from build123d import *

# Parameters (mm, degrees)
SKETCH_1_R          = 1.5000000000000002
EXTRUDE_1_DEPTH     = 10
EXTRUDE_START       = 1
SKETCH_2_R          = 2.75
SKETCH_2_R_2        = 1.5000000000000002
EXTRUDE_2_DEPTH     = 1
SKETCH_3_R          = 2.75
SKETCH_3_R_2        = 1.5000000000000002
EXTRUDE_3_DEPTH     = 1
SKETCH_5_R          = 6.5
EXTRUDE_4_DEPTH     = 18
SKETCH_7_R          = 4.499999999999999
CUT_EXTRUDE_1_DEPTH = 18
SKETCH_9_R          = 2.8700119692288277
SKETCH_12_W         = 5.249259279764373
SKETCH_12_H         = 2.7755664511126334
SKETCH_12_H_2       = 2.7755664511126383
EXTRUDE_5_DEPTH     = 5
CUT_EXTRUDE_2_DEPTH = 20


with BuildPart() as part:
    # 草图1 → 凸台-拉伸1 (new body)
    with BuildSketch(Plane.XY):
        with BuildLine():
            Line((-2.75, 0), (-2.7500000000000004, 9.5))
            Line((-2.7500000000000004, 9.5), (2.7500000000000004, 9.5))
            Line((2.7500000000000004, 9.5), (2.75, 0))
            ThreePointArc((2.75, 0), (-5.1e-16, -2.75), (-2.75, 0))
        make_face()
        Circle(SKETCH_1_R, mode=Mode.SUBTRACT)
    extrude(amount=EXTRUDE_1_DEPTH)

    # 草图2 → 凸台-拉伸2 (add)
    with BuildSketch(Plane(origin=(0, 0, 0), x_dir=(-1, 0, 0), z_dir=(0, 0, -1)).offset(EXTRUDE_START)):
        Circle(SKETCH_2_R)
        Circle(SKETCH_2_R_2, mode=Mode.SUBTRACT)
    extrude(amount=-EXTRUDE_2_DEPTH)

    # 草图3 → 凸台-拉伸3 (add)
    with BuildSketch(Plane.XY.offset(10)):
        with Locations(Location((0, 0, 0), (0, 0, 180))):
            Circle(SKETCH_3_R)
        with Locations(Location((0, 0, 0), (0, 0, 180))):
            Circle(SKETCH_3_R_2, mode=Mode.SUBTRACT)
    extrude(amount=EXTRUDE_3_DEPTH)

    # 草图5 → 凸台-拉伸4 (add)
    with BuildSketch(Plane.ZY.offset(4.75)):
        with Locations(Location((5, 13.164932727725386, 0), (0, 0, 270))):
            Circle(SKETCH_5_R)
    extrude(amount=-EXTRUDE_4_DEPTH)

    # 草图7 → 切除-拉伸1 (cut)
    with BuildSketch(Plane.ZY.offset(4.75)):
        with Locations(Location((5, 13.164932727725386, 0), (0, 0, 270))):
            Circle(SKETCH_7_R)
    extrude(amount=-CUT_EXTRUDE_1_DEPTH, mode=Mode.SUBTRACT)

    # 扫描2: sweep along a path in 草图11
    with BuildLine(Plane(origin=(0, 0, 5), x_dir=(-1, 0, 0), z_dir=(0, 0, -1))) as sweep_2_path:
        Line((-7, 24), (0, 19))
    # 草图9 → 扫描2 (sweep)
    with BuildSketch(Plane(origin=(0, 19, 0), x_dir=(1, 0, 0), z_dir=(0, 1, 0))):
        with Locations((-0.00737750074134282, -4.885467390073623)):
            Circle(SKETCH_9_R)
    sweep(path=sweep_2_path.line)

    # 草图12 → 凸台-拉伸5 (add)
    with BuildSketch(Plane(origin=(0, 19, 0), x_dir=(1, 0, 0), z_dir=(0, 1, 0))):
        with Locations((9.375370360117813, -3.6122167744436835)):
            Rectangle(SKETCH_12_W, SKETCH_12_H)
        with Locations((9.375370360117813, -6.387783225556319)):
            Rectangle(SKETCH_12_W, SKETCH_12_H_2)
    extrude(amount=EXTRUDE_5_DEPTH)

    # 草图13 → 旋转1 (revolve)
    with BuildSketch(Plane(origin=(0, 0, 5), x_dir=(-1, 0, 0), z_dir=(0, 0, -1)), mode=Mode.PRIVATE) as revolve_1_sk:
        with BuildLine():
            Line((-7.006191849278699, 24), (-5.006191849278698, 24))
            Line((-5.006191849278698, 24), (-5.912975516058456, 25.133479583474696))
            ThreePointArc((-5.912975516058456, 25.133479583474696), (-5.354842290747966, 27.079262147512125), (-7.006191849278699, 28.25))
            Line((-7.006191849278699, 28.25), (-7.006191849278698, 26.5))
            Line((-7.006191849278698, 26.5), (-7.006191849278699, 24))
        make_face()
    revolve(revolve_1_sk.sketch.rotate(Axis((7.006191849278698, 26.5, 5), (5e-16, 1, 0)), 180), axis=Axis((7.006191849278698, 26.5, 5), (5e-16, 1, 0)))

    # 草图14 → 切除-拉伸2 (cut, symmetric)
    with BuildSketch(Plane(origin=(0, 0, 5), x_dir=(-1, 0, 0), z_dir=(0, 0, -1))):
        with BuildLine():
            Line((-13.5, 19), (-13.5, 6.499999999999999))
            Line((-13.5, 6.499999999999999), (-6.000000000000001, 6.499999999999999))
            add(Edge.make_bspline(
                [(-13.5, 19), (-11.192290817282267, 18.56878443157226), (-8.111749647069864, 14.147051950991559), (-6.7530537895194716, 9.319622020478048), (-6.000000000000001, 6.499999999999999)],
                knots=[0, 0, 0, 0, 0.42648903061023624, 1, 1, 1, 1], degree=3))
        make_face()
    extrude(amount=CUT_EXTRUDE_2_DEPTH, both=True, mode=Mode.SUBTRACT)


solid = part.part
Here's how the part is built. I have some questions about the finished solid (model axes, mm). A direction names the side the tool comes from. Give positions to 0.01 mm unless a question says otherwise; leave off trailing zeros. Order: outer loops, then holes, each group sorted by start corner. A loop starts at its lowest first (then second) coordinate and runs counter-clockwise, first axis right, second up. Notation, with made-up numbers: (-25, -17.75) -> (25, -17.75) arc R20 ccw to (25, 21.25) -> close; hole circle Ø3 at (-26, 83). An arc over 180 degrees is marked (long way). One line per item, written item: value. Start each with the question number.
1. We'd pull the mould along Y, two halves only. Please class faces 1 (the face through (9, 24, 4)), 2 (the face through (9, 21, 2.224)), 3 (the face through (9, 21, 7.776)): released by +Y, released by -Y, zero draft, split by the parting line, or undercut.
2. Imagine slicing it at A-A, the plane y = 2. List the corners of the cut face in (x, z) for me, plus the area to 4 significant figures.
3. For faces 4 (the face through (1.24, 17.66, 5.2)), 5 (the face through (-1.2, -1.2, -1)), 6 (the face through (-1.2, 1.2, 11)), which set-ups out of +Z, -Z, +X, -X, +Y, -Y let a thin tool reach every point of the face, with its end or its side?
4. Imagine slicing it at D-D, the plane y = 5.5. List the corners of the cut face in (x, z) for me.
5. Will these pins go through, and if not, where does the flat tip stop? pin 1 Ø1.5 at (x, z) = (-2.5, 4) entering from +Y; pin 2 Ø4 at (y, z) = (22.5, 3.5) entering from +X; pin 3 Ø4 at (x, z) = (1, 8.5) entering from -Y; pin 4 Ø1.5 at (x, z) = (4, 7.5) entering from -Y.
6. I need wall thicknesses on probe 1 along Y at (x, z) = (-1, 4.25); probe 2 along Y at (x, z) = (4.5, 7.25); probe 3 along X at (y, z) = (0.5, 7.75). Which ranges of each line are inside material? Lowest first, please. Write a range as from..to.
7. Imagine slicing it at B-B, the plane z = 8.5. Count the separate pieces of the cut face and the enclosed holes in it, plus the area to 3 significant figures.
Values follow:
1. face 1: released by +Y
1. face 2: undercut
1. face 3: zero draft
2. outline: (-2.75, 0) -> (-1.89, 0) -> (-1.89, -1) -> (1.89, -1) -> (1.89, 0) -> (2.75, 0) -> (2.75, 10) -> (1.89, 10) -> (1.89, 11) -> (-1.89, 11) -> (-1.89, 10) -> (-2.75, 10) -> close
2. area: 62.55 mm2
3. face 4: +X, -X
3. face 5: -Z, +X, -X, -Y
3. face 6: +Z, +X, -X, -Y
4. outline: (-2.75, 0) -> (2.75, 0) -> (2.75, 10) -> (-2.75, 10) -> close
5. pin 1: stops at y = 19.73
5. pin 2: stops at x = 12
5. pin 3: stops at y = -2.75
5. pin 4: stops at y = 6.9
6. probe 1: y = -2.56..-1.12, 1.12..8.73, 17.6..20.29
6. probe 2: y = 7.07..9.27, 17.06..19.26, 21.06..23.38
6. probe 3: x = -2.75..-1.41, 1.41..2.75
7. separate pieces: 2
7. enclosed holes: 1
7. area: 118 mm2
